```python
from build123d import *

# Parameters (mm, degrees)
F1_DEPTH    = 10
F3_D        = 10
F3_DEPTH    = 100
F3_TIP      = 3.0043030951
F5_DEPTH    = 25
F6_T1_DEPTH = 10


# Not quite as in the source:
# - a fillet or chamfer that OpenCascade refuses, or shapes differently, is made with other operations: its cross-section is extruded or revolved along the edge and cut away or added


with BuildPart() as f1:
    # F0 (on Right) → F1 (new body)
    with BuildSketch(Plane.YZ):
        Polygon((0, 150), (0, 0), (100, 0), (100, 100), (100, 200), (0, 200), align=None)
        Polygon((-45, 200), (0, 150), (0, 200), (100, 200), (100, 100), (160, 130), (135, 230), align=None)
    extrude(amount=F1_DEPTH)

    # F3
    with Locations(Plane.YZ.offset(10)):
        with Locations((25, 120), (75, 120)):
            Hole(F3_D / 2, depth=F3_DEPTH)
            with Locations((0, 0, -(F3_DEPTH + F3_TIP / 2))):  # 118° drill point
                Cone(0, F3_D / 2, F3_TIP, mode=Mode.SUBTRACT)

    # F4 (on face) → F5 (cut)
    with BuildSketch(Plane.YZ.offset(10)):
        with BuildLine():
            Line((0, 0), (50, 0))
            ThreePointArc((50, 0), (36.033388833, 42.8809920236), (0, 70))
            Line((0, 70), (0, 0))
        make_face()
    extrude(amount=-F5_DEPTH, mode=Mode.SUBTRACT)

    # F6: fillet of radius 150 on 1 edges, made by hand

    # F6_s2 → F6_t1 (join)
    with BuildSketch(Plane.YZ):
        with BuildLine():
            ThreePointArc((160, 130), (115.83592135, 77.082039325), (100, 10))
            Line((100, 10), (100, 100))
            Line((100, 100), (160, 130))
        make_face()
    extrude(amount=F6_T1_DEPTH)


solid = f1.part
```
Geometry check sheet. Reference: the model listing, model coordinates, mm. A direction names the side the tool comes from. Give positions to 0.01 mm unless a question says otherwise; leave off trailing zeros. Write each loop counter-clockwise with the first axis right and the second up, starting at its lowest first coordinate (ties: lowest second). Pieces come first, ordered by that corner, then holes. Notation, with made-up numbers: (-6.75, 13.25) -> (10.25, 13.25) arc R24 cw to (10.25, 30.25) -> close; hole circle Ø9 at (13.25, 10). An arc over 180 degrees is marked (long way). One line per question, with ' | ' between items.
Item 1: Depth check by flat-ended pin: pin 1 (4 mm diameter, centred on x = 4.5, y = 27, fed in from +Z); pin 2 (6 mm diameter, centred on x = 4, z = 179, fed in from +Y); pin 3 (13 mm diameter, centred on y = 75, z = 120, fed in from +X); pin 4 (1.5 mm diameter, centred on x = 7.5, y = 3, fed in from -Z). Enter the tip coordinate at first touch or a pass-through.
Determined:
pin 1: z = 212.33 | pin 2: y = 148.5 | pin 3: x = 10 | pin 4: z = 68.56
Item 2: Scan lines: line 1 along Y through (x, z) = (1, 121.5); line 2 along Z through (x, y) = (5.5, 75); line 3 along Z through (x, y) = (7.75, 25). Record each from-to range of solid material in increasing order.
Determined:
line 1: 0 to 20.23, 29.77 to 70.23, 79.77 to 149.66 | line 2: 0 to 115, 125 to 220 | line 3: 55.19 to 115, 125 to 211.67
Item 3: Sectioned sample at B-B, the plane x = 6.25. Record the boundary of the cut face in (y, z), plus the area to 3 significant figures.
Determined:
outline: (-45, 200) -> (0, 150) -> (0, 70) arc R75 cw to (50, 0) -> (100, 0) -> (100, 10) arc R150 cw to (160, 130) -> (135, 230) -> close; hole circle Ø10 at (25, 120); hole circle Ø10 at (75, 120) | area: 27,000 mm^2
Item 4: Sectioned sample at D-D, the plane y = 25. Record the boundary of the cut face in (x, z), plus the area to 3 significant figures.
Determined:
outline: (0, 55.19) -> (10, 55.19) -> (10, 115) -> (0, 115) -> close; (0, 125) -> (10, 125) -> (10, 211.67) -> (0, 211.67) -> close | area: 1,460 mm^2
Item 5: Sectioned sample at C-C, the plane z = 120. Record the boundary of the cut face in (x, y).
Determined:
outline: (0, 0) -> (10, 0) -> (10, 20) -> (0, 20) -> close; (0, 30) -> (10, 30) -> (10, 70) -> (0, 70) -> close; (0, 80) -> (10, 80) -> (10, 148.02) -> (0, 148.02) -> close
Item 6: Draft check along Z on faces 4 (the flat face through (4.93, -22.815, 175.35)), 5 (the cylindrical face through (5, 30, 120)), 6 (the flat face through (4.93, 46.26, 215.21)). Enter one of: released by +Z, released by -Z, zero draft, split by the parting line, or undercut.
Determined:
face 4: released by -Z | face 5: undercut | face 6: released by +Z
Item 7: Sectioned sample at A-A, the plane y = 75. Record the boundary of the cut face in (x, z), plus the area to 3 significant figures.
Determined:
outline: (0, 0) -> (10, 0) -> (10, 115) -> (0, 115) -> close; (0, 125) -> (10, 125) -> (10, 220) -> (0, 220) -> close | area: 2,100 mm^2
Item 8: Access from +Z, -Z, +X, -X, +Y, -Y to the whole of each face (thin tool, end or side, straight path). Record for faces 1 (the flat face through (5, 0, 111)), 2 (the flat face through (5, 100, 5)), 3 (the cylindrical face through (4.93, 70.381, 118.085)).
Determined:
face 1: -Z, +X, -X, -Y | face 2: -Z, +X, -X, +Y | face 3: +X, -X
